from build123d import *

# Parameters (mm, degrees)
BOSS_EXTRUDE1_DEPTH = 25
SKETCH5_R           = 2.5
CUT_EXTRUDE4_DEPTH  = 90
CHAMFER1_SIZE       = 2.7


with BuildPart() as part:
    # Sketch1 → Boss-Extrude1 (new, symmetric)
    with BuildSketch(Plane.XY):
        with BuildLine():
            Line((-10, -9.124404748), (-19, -9.124404748))
            Line((-19, -9.124404748), (-19, -23.124404748))
            Line((-19, -23.124404748), (32, -23.124404748))
            Line((32, -23.124404748), (32, 27.875595252))
            Line((32, 27.875595252), (25, 27.875595252))
            Line((25, 27.875595252), (25, -9.124404748))
            Line((25, -9.124404748), (10, -9.124404748))
            ThreePointArc((10, -9.124404748), (12.023420987, -16.574878268), (6.509119733, -11.171520993))
            ThreePointArc((6.509119733, -11.171520993), (0, -13), (-6.509119733, -11.171520993))
            ThreePointArc((-6.509119733, -11.171520993), (-12.023420987, -16.574878268), (-10, -9.124404748))
        make_face()
    extrude(amount=BOSS_EXTRUDE1_DEPTH, both=True)

    # Sketch5 → Cut-Extrude4 (cut)
    with BuildSketch(Plane(origin=(32, 0, 0), x_dir=(0, 0, -1), z_dir=(1, 0, 0))):
        with Locations(Location((17, -2.724404748, 0), (0, 0, 90))):
            Circle(SKETCH5_R)
        with Locations(Location((17, 22.275595252, 0), (0, 0, 90))):
            Circle(SKETCH5_R)
        with Locations(Location((-17, -2.724404748, 0), (0, 0, 90))):
            Circle(SKETCH5_R)
        with Locations(Location((-17, 22.275595252, 0), (0, 0, 90))):
            Circle(SKETCH5_R)
    extrude(amount=-CUT_EXTRUDE4_DEPTH, mode=Mode.SUBTRACT)

    # Chamfer1
    chamfer1_edges = [part.edges().sort_by_distance(p)[0] for p in [
        (25, 19.775595252, -17),
        (25, -5.224404748, 17),
        (25, 19.775595252, 17),
        (25, -5.224404748, -17),
    ]]
    chamfer(chamfer1_edges, length=CHAMFER1_SIZE)


solid = part.part
Can you work these out from the model? Positions are in its coordinate system, mm. A direction names the side the tool comes from. Round coordinates to 2 decimals unless told otherwise and drop trailing zeros. Write each loop counter-clockwise with the first axis right and the second up, starting at its lowest first coordinate (ties: lowest second). Pieces come first, ordered by that corner, then holes. Notation, with made-up numbers: M 51.25,1.25 L 75.25,1.25 A23 cw 75.25,9.25 Z; hole C 77,-21.75 d9. An arc over 180 degrees is marked long. Use CSV: the item, a comma, the result in double quotes.
(1) We'd pull the mould along Y, two halves only. Please class faces 1 (the flat face through (16, -11, 25)), 2 (the flat face through (6, -23.124, 0)), 3 (the cylindrical face through (-11.896, -16.647, 0.35)), 4 (the cylindrical face through (29.88, 20.29, -18.52)): +Y half, -Y half, draft (parallel to the pull), parting line (faces both ways), or undercut.
Check values:
face 1,"draft"
face 2,"-Y half"
face 3,"undercut"
face 4,"undercut"
(2) On a 3-axis mill with a long thin cutter (end or side, diameter ignored), from which of +Z, -Z, +X, -X, +Y, -Y can I reach the whole of each face in a straight line? I mean faces 5 (the flat face through (18, -9.124, 0)), 6 (the flat face through (32, 2, 0)). Say none if no direction works.
Check values:
face 5,"+Z, -Z, -X, +Y"
face 6,"+Z, -Z, +X, +Y, -Y"
(3) Imagine slicing it at C-C (z = 0.5). Write out the boundary of the cut face in (x, y).
Check values:
outline,"M -19,-23.12 L 32,-23.12 L 32,27.88 L 25,27.88 L 25,-9.12 L 10,-9.12 A4 cw long 6.51,-11.17 A12.5 cw -6.51,-11.17 A4 cw long -10,-9.12 L -19,-9.12 Z"
(4) I'm going to push flat-ended pins straight in: pin 1 (10 mm diameter, centred on y = -3, z = -18.5, fed in from -X); pin 2 (6 mm diameter, centred on x = -8, z = -17, fed in from +Y); pin 3 (1 mm diameter, centred on x = 11, y = -8.5, fed in from -Z); pin 4 (8 mm diameter, centred on x = -4, z = -5, fed in from +Y). Where does each tip first touch, or does it pass through?
Check values:
pin 1,"x = 25"
pin 2,"y = -9.12"
pin 3,"through"
pin 4,"y = -11.17"
(5) Imagine slicing it at D-D (x = 20). Write out the boundary of the cut face in (y, z).
Check values:
outline,"M -23.12,-25 L -9.12,-25 L -9.12,25 L -23.12,25 Z"
(6) Imagine slicing it at B-B (x = -13). Write out the boundary of the cut face in (y, z).
Check values:
outline,"M -23.12,-25 L -15.77,-25 L -15.77,25 L -23.12,25 Z; M -10.48,-25 L -9.12,-25 L -9.12,25 L -10.48,25 Z"
(7) I need wall thicknesses on line 1 along Y through (x, z) = (-15, 7); line 2 along X through (y, z) = (0.5, -3.5); line 3 along Y through (x, z) = (13.5, -5.5). Which ranges of each line are inside material? Lowest first, please.
Check values:
line 1,"-23.12 to -9.12"
line 2,"25 to 32"
line 3,"-23.12 to -15.06, -11.19 to -9.12"
(8) Imagine slicing it at A-A (z = 17). Write out the boundary of the cut face in (x, y).
Check values:
outline,"M -19,-23.12 L 32,-23.12 L 32,-5.22 L 27.7,-5.22 L 25,-7.92 L 25,-9.12 L 10,-9.12 A4 cw long 6.51,-11.17 A12.5 cw -6.51,-11.17 A4 cw long -10,-9.12 L -19,-9.12 Z; M 25,2.48 L 27.7,-0.22 L 32,-0.22 L 32,19.78 L 27.7,19.78 L 25,17.08 Z; M 25,27.48 L 27.7,24.78 L 32,24.78 L 32,27.88 L 25,27.88 Z"
